Autodesk Inventor part; units mm, degrees
ref_plane "YZ Plane" through (0, 0, 0) normal (1, 0, 0) x (0, 1, 0)
ref_plane "XZ Plane" through (0, 0, 0) normal (0, 1, 0) x (-1, 0, 0)
ref_plane "XY Plane" through (0, 0, 0) normal (0, 0, 1) x (1, 0, 0)
sketch "Skizze1" plane through (0, 0, 0) normal (0, 0, 1) x (1, 0, 0)
  line L0 (-29.2, 4.2) -> (29.2, 4.2)
  line L1 (29.2, 4.2) -> (29.2, -5.8)
  line L2 (29.2, -5.8) -> (31, -5.8)
  line L3 (31, -5.8) -> (31, -56.6)
  line L4 (31, -56.6) -> (-31, -56.6)
  line L5 (-31, -56.6) -> (-31, -5.8)
  line L6 (-31, -5.8) -> (-29.2, -5.8)
  line L7 (-29.2, -5.8) -> (-29.2, 4.2)
  line L8 (-43.4, 0) -> (43.4, 0)
  line L9 (0, 16.36) -> (0, -68.76)
  point P0 (0, 0)
  dimension "d0" = 4.2
  dimension "d1" = 5.8
  dimension "d2" = 56.6
  dimension "d3" = 62
  dimension "d4" = 58.4
extrude "Extrusion1" add sketch "Skizze1" along normal blind 1.6
sketch "Skizze2" plane through (0, 0, 1.6) normal (0, 0, 1) x (1, 0, 0)
  line L0 (-28, -53.6) -> (28, -53.6) construction
  line L1 (0, 16.36) -> (0, -68.76) construction
  line L2 (-43.4, 0) -> (43.4, 0) construction
  point P0 (0, 0)
  dimension "d7" = 53.6
  dimension "d8" = 56
hole "Bohrung1" at (-28, -53.6, 1.6) at (28, -53.6, 1.6) direction (0, 0, -1) diameter 3.2 end through all
sketch "Skizze3" plane through (0, 0, 1.6) normal (0, 0, 1) x (1, 0, 0)
  line L0 (0, 16.36) -> (0, -68.76)
  line L1 (-43.4, 0) -> (43.4, 0)
  line L2 (-30, -6.2) -> (30, -6.2)
  line L3 (30, -6.2) -> (30, -49.2)
  line L4 (30, -49.2) -> (-30, -49.2)
  line L5 (-30, -49.2) -> (-30, -6.2)
  point P0 (0, 0)
  dimension "d16" = 60
  dimension "d17" = 43
  dimension "d18" = 6.2
extrude "Extrusion2" add sketch "Skizze3" along normal blind 4
shell "Wandung1" thickness 4 removed faces 1 at (10, -20.5333, 5.6)
properties part number "LT24" material "Phenolharz"
Here's how the part is built. I have some questions about the finished solid (model axes, mm). A direction names the side the tool comes from. Round coordinates to 2 decimals unless told otherwise and drop trailing zeros. Order: outer loops, then holes, each group sorted by start corner. A loop starts at its lowest first (then second) coordinate and runs counter-clockwise, first axis right, second up. Notation, with made-up numbers: (-26.5, 73.5) -> (-8.5, 73.5) arc R9 ccw to (-8.5, 90.5) -> close; hole circle Ø11 at (54.25, 52.5). An arc over 180 degrees is marked (long way). Use a Markdown table: item, result. Add a question column.
(1) For pin 1 Ø10.5 at (x, y) = (0.5, -31) entering from +Z; pin 2 Ø3 at (x, z) = (8, 4.5) entering from +Y; pin 3 Ø1.5 at (x, z) = (17, 2.5) entering from -Y; pin 4 Ø3 at (x, y) = (-9.5, -29.5) entering from -Z, each with a flat end and sliding along its axis, tell me the tip position at first contact or that it passes through.
(2) For faces 1 (the face through (0, -49.2, 4)), 2 (the face through (-30, -28, 4)), 3 (the face through (0, -10.2, 5)), 4 (the face through (30, -27, 4)), which set-ups out of +Z, -Z, +X, -X, +Y, -Y let a thin tool reach every point of the face, with its end or its side?
(3) If we mould it in two halves opening along Y, with no side actions, what happens to faces 5 (the face through (0, 4.2, 1)), 6 (the face through (0, -47, 5.6)), 7 (the face through (26.414, -53.392, 0.789))? For each: released by +Y, released by -Y, zero draft, split by the parting line, or undercut.
(4) Suppose I cut it at C-C, the plane x = -28. Please give me the cut outline in (y, z), and give its area (3 significant figures).
(5) I need wall thicknesses on line 1 along X through (y, z) = (-53.6, 0.8); line 2 along Y through (x, z) = (-12.5, 4.85); line 3 along X through (y, z) = (-37, 4.95). Which ranges of each line are inside material? Lowest first, please.
(6) Suppose I cut it at A-A, the plane y = -53.6. Please give me the cut outline in (x, z).
(7) Suppose I cut it at B-B, the plane x = -16.5. Please give me the cut outline in (y, z), and give its area (3 significant figures).
(8) Suppose I cut it at D-D, the plane y = -22. Please give me the cut outline in (x, z).
Verdict:
| question | item | result |
|---|---|---|
| 1 | pin 1 | z = 4 |
| 1 | pin 2 | y = -6.2 |
| 1 | pin 3 | y = -49.2 |
| 1 | pin 4 | z = 0 |
| 2 | face 1 | +Z, +X, -X, -Y |
| 2 | face 2 | +Z, -X, +Y, -Y |
| 2 | face 3 | +Z |
| 2 | face 4 | +Z, +X, +Y, -Y |
| 3 | face 5 | released by +Y |
| 3 | face 6 | zero draft |
| 3 | face 7 | undercut |
| 4 | outline | (-56.6, 0) -> (-55.2, 0) -> (-55.2, 1.6) -> (-56.6, 1.6) -> close; (-52, 0) -> (4.2, 0) -> (4.2, 1.6) -> (-6.2, 1.6) -> (-6.2, 5.6) -> (-49.2, 5.6) -> (-49.2, 1.6) -> (-52, 1.6) -> close |
| 4 | area | 264 mm2 |
| 5 | line 1 | -31 to -29.6, -26.4 to 26.4, 29.6 to 31 |
| 5 | line 2 | -49.2 to -45.2, -10.2 to -6.2 |
| 5 | line 3 | -30 to -26, 26 to 30 |
| 6 | outline | (-31, 0) -> (-29.6, 0) -> (-29.6, 1.6) -> (-31, 1.6) -> close; (-26.4, 0) -> (26.4, 0) -> (26.4, 1.6) -> (-26.4, 1.6) -> close; (29.6, 0) -> (31, 0) -> (31, 1.6) -> (29.6, 1.6) -> close |
| 7 | outline | (-56.6, 0) -> (4.2, 0) -> (4.2, 1.6) -> (-6.2, 1.6) -> (-6.2, 5.6) -> (-10.2, 5.6) -> (-10.2, 4) -> (-45.2, 4) -> (-45.2, 5.6) -> (-49.2, 5.6) -> (-49.2, 1.6) -> (-56.6, 1.6) -> close |
| 7 | area | 213 mm2 |
| 8 | outline | (-31, 0) -> (31, 0) -> (31, 1.6) -> (30, 1.6) -> (30, 5.6) -> (26, 5.6) -> (26, 4) -> (-26, 4) -> (-26, 5.6) -> (-30, 5.6) -> (-30, 1.6) -> (-31, 1.6) -> close |
